Design review of the part built by this model. Coordinates are the model's own, in mm. A direction names the side the tool comes from. Give positions to 0.01 mm unless a question says otherwise; leave off trailing zeros. Loops run counter-clockwise (first coordinate to the right, second up) from the corner with the lowest first, then second, coordinate; pieces in that order, holes last. Notation, with made-up numbers: (2.25, 7.25) - (36.25, 7.25) arc R32 cw to (36.25, 42.25) - close; hole circle Ø10 at (-5, -39). An arc over 180 degrees is marked (long way). Write each question's results on one line, items separated by ' | '.
```python
from build123d import *

# Parameters (mm, degrees)
SKETCH1_W            = 31
SKETCH1_H            = 29
BOSS_EXTRUDE1_DEPTH  = 1
SKETCH2_W            = 7
SKETCH2_H            = 8
BOSS_EXTRUDE2_DEPTH  = 13
SKETCH3_W            = 7
SKETCH3_H            = 7
BOSS_EXTRUDE3_DEPTH  = 5
SKETCH4_W            = 4
SKETCH4_H            = 4
BOSS_EXTRUDE4_DEPTH  = 5
SKETCH5_R            = 2.75
CUT_EXTRUDE1_DEPTH   = 8
SKETCH6_W            = 1.591238362
SKETCH6_H            = 3.57435367
BOSS_EXTRUDE5_DEPTH  = 0.1
SKETCH7_R            = 0.879599875
BOSS_EXTRUDE6_DEPTH  = 8
FILLET2_R            = 0.5
SKETCH8_W            = 7.71
SKETCH8_H            = 5.14
BOSS_EXTRUDE7_DEPTH  = 1.5
SKETCH9_W            = 1
SKETCH9_H            = 1
BOSS_EXTRUDE8_DEPTH  = 4
SKETCH10_W           = 0.8
SKETCH10_H           = 1.5
BOSS_EXTRUDE9_DEPTH  = 0.5
SKETCH11_W           = 5
SKETCH11_H           = 4
BOSS_EXTRUDE10_DEPTH = 2
SKETCH12_W           = 0.6
SKETCH12_H           = 2.642715267
BOSS_EXTRUDE11_DEPTH = 0.5
SKETCH13_W           = 2.5
SKETCH13_H           = 2
BOSS_EXTRUDE12_DEPTH = 0.5
SKETCH14_W           = 2.401106116
SKETCH14_H           = 1.2192983
BOSS_EXTRUDE13_DEPTH = 1


with BuildPart() as part:
    # Sketch1 → Boss-Extrude1 (new body)
    with BuildSketch(Plane(origin=(0, 0, 0), x_dir=(1, 0, 0), z_dir=(0, 1, 0))):
        with Locations((15.5, 14.5)):
            Rectangle(SKETCH1_W, SKETCH1_H)
    extrude(amount=BOSS_EXTRUDE1_DEPTH)

    # Sketch2 → Boss-Extrude2 (add)
    with BuildSketch(Plane.ZY):
        with Locations((-5.5, 4)):
            Rectangle(SKETCH2_W, SKETCH2_H)
    extrude(amount=-BOSS_EXTRUDE2_DEPTH)

    # Sketch3 → Boss-Extrude3 (add)
    with BuildSketch(Plane(origin=(0, 1, 0), x_dir=(1, 0, 0), z_dir=(0, 1, 0))):
        with Locations((6.5, 13.5)):
            Rectangle(SKETCH3_W, SKETCH3_H)
    extrude(amount=BOSS_EXTRUDE3_DEPTH)

    # Sketch4 → Boss-Extrude4 (add)
    with BuildSketch(Plane(origin=(0, 6, 0), x_dir=(1, 0, 0), z_dir=(0, 1, 0))):
        with Locations((6.5, 13.5)):
            Rectangle(SKETCH4_W, SKETCH4_H)
    extrude(amount=BOSS_EXTRUDE4_DEPTH)

    # Sketch5 → Cut-Extrude1 (cut)
    with BuildSketch(Plane.ZY):
        with Locations((-5.5, 4.5)):
            Circle(SKETCH5_R)
    extrude(amount=-CUT_EXTRUDE1_DEPTH, mode=Mode.SUBTRACT)

    # Sketch6 → Boss-Extrude5 (add)
    with BuildSketch(Plane.XY.offset(-2)):
        with Locations((10.684219388, 2.787176835)):
            Rectangle(SKETCH6_W, SKETCH6_H)
    extrude(amount=BOSS_EXTRUDE5_DEPTH)

    # Sketch7 → Boss-Extrude6 (add)
    with BuildSketch(Plane.ZY.offset(-8)):
        with Locations((-5.5, 4.5)):
            Circle(SKETCH7_R)
    extrude(amount=BOSS_EXTRUDE6_DEPTH)

    # Fillet2
    fillet2_edges = [part.edges().sort_by_distance(p)[0] for p in [
        (0, 4.5, -6.379599875),
    ]]
    fillet(fillet2_edges, radius=FILLET2_R)

    # Sketch8 → Boss-Extrude7 (add)
    with BuildSketch(Plane(origin=(0, 1, 0), x_dir=(1, 0, 0), z_dir=(0, 1, 0))):
        with Locations((15.495, 24.43)):
            Rectangle(SKETCH8_W, SKETCH8_H)
        with Locations((6.785, 24.43)):
            Rectangle(SKETCH8_W, SKETCH8_H)
        with Locations((24.205, 24.43)):
            Rectangle(SKETCH8_W, SKETCH8_H)
    extrude(amount=BOSS_EXTRUDE7_DEPTH)

    # Sketch9 → Boss-Extrude8 (add)
    with BuildSketch(Plane(origin=(0, 2.5, 0), x_dir=(1, 0, 0), z_dir=(0, 1, 0))):
        with Locations((6.971468334, 25.685)):
            Rectangle(SKETCH9_W, SKETCH9_H)
        with Locations((4.431468334, 25.685)):
            Rectangle(SKETCH9_W, SKETCH9_H)
        with Locations((9.511468334, 25.685)):
            Rectangle(SKETCH9_W, SKETCH9_H)
        with Locations((4.431468334, 23.145)):
            Rectangle(SKETCH9_W, SKETCH9_H)
        with Locations((13.051468334, 23.145)):
            Rectangle(SKETCH9_W, SKETCH9_H)
        with Locations((6.971468334, 23.145)):
            Rectangle(SKETCH9_W, SKETCH9_H)
        with Locations((9.511468334, 23.145)):
            Rectangle(SKETCH9_W, SKETCH9_H)
        with Locations((18.131468334, 25.685)):
            Rectangle(SKETCH9_W, SKETCH9_H)
        with Locations((18.131468334, 23.145)):
            Rectangle(SKETCH9_W, SKETCH9_H)
        with Locations((15.591468334, 23.145)):
            Rectangle(SKETCH9_W, SKETCH9_H)
        with Locations((15.591468334, 25.685)):
            Rectangle(SKETCH9_W, SKETCH9_H)
        with Locations((13.051468334, 25.685)):
            Rectangle(SKETCH9_W, SKETCH9_H)
        with Locations((21.671468334, 23.145)):
            Rectangle(SKETCH9_W, SKETCH9_H)
        with Locations((26.751468334, 25.685)):
            Rectangle(SKETCH9_W, SKETCH9_H)
        with Locations((26.751468334, 23.145)):
            Rectangle(SKETCH9_W, SKETCH9_H)
        with Locations((24.211468334, 23.145)):
            Rectangle(SKETCH9_W, SKETCH9_H)
        with Locations((24.211468334, 25.685)):
            Rectangle(SKETCH9_W, SKETCH9_H)
        with Locations((21.671468334, 25.685)):
            Rectangle(SKETCH9_W, SKETCH9_H)
    extrude(amount=BOSS_EXTRUDE8_DEPTH)

    # Sketch10 → Boss-Extrude9 (add)
    with BuildSketch(Plane(origin=(0, 1, 0), x_dir=(1, 0, 0), z_dir=(0, 1, 0))):
        with Locations((18.786083485, 18.300770285)):
            Rectangle(SKETCH10_W, SKETCH10_H)
        with Locations((14.786083485, 18.300770285)):
            Rectangle(SKETCH10_W, SKETCH10_H)
        with Locations((22.786083485, 18.300770285)):
            Rectangle(SKETCH10_W, SKETCH10_H)
        with Locations((26.786083485, 18.300770285)):
            Rectangle(SKETCH10_W, SKETCH10_H)
    extrude(amount=BOSS_EXTRUDE9_DEPTH)

    # Sketch11 → Boss-Extrude10 (add)
    with BuildSketch(Plane(origin=(0, 1, 0), x_dir=(1, 0, 0), z_dir=(0, 1, 0))):
        with Locations((25.443805994, 10.374755585)):
            Rectangle(SKETCH11_W, SKETCH11_H)
        with Locations((18.443805994, 10.374755585)):
            Rectangle(SKETCH11_W, SKETCH11_H)
    extrude(amount=BOSS_EXTRUDE10_DEPTH)

    # Sketch12 → Boss-Extrude11 (add)
    with BuildSketch(Plane(origin=(0, 1, 0), x_dir=(1, 0, 0), z_dir=(0, 1, 0))):
        with Locations((17.095277575, 13.696113219)):
            Rectangle(SKETCH12_W, SKETCH12_H)
        with Locations((24.095277575, 13.696113219)):
            Rectangle(SKETCH12_W, SKETCH12_H)
        with Locations((18.365277575, 13.696113219)):
            Rectangle(SKETCH12_W, SKETCH12_H)
        with Locations((19.635277575, 13.696113219)):
            Rectangle(SKETCH12_W, SKETCH12_H)
        with Locations((25.365277575, 13.696113219)):
            Rectangle(SKETCH12_W, SKETCH12_H)
        with Locations((26.635277575, 13.696113219)):
            Rectangle(SKETCH12_W, SKETCH12_H)
    extrude(amount=BOSS_EXTRUDE11_DEPTH)

    # Sketch13 → Boss-Extrude12 (add)
    with BuildSketch(Plane(origin=(0, 1, 0), x_dir=(1, 0, 0), z_dir=(0, 1, 0))):
        with Locations((18.365277575, 7.374755585)):
            Rectangle(SKETCH13_W, SKETCH13_H)
        with Locations((25.365277575, 7.374755585)):
            Rectangle(SKETCH13_W, SKETCH13_H)
    extrude(amount=BOSS_EXTRUDE12_DEPTH)

    # Sketch14 → Boss-Extrude13 (add)
    with BuildSketch(Plane(origin=(0, 1, 0), x_dir=(1, 0, 0), z_dir=(0, 1, 0))):
        with Locations((23.540566393, 4.488126974)):
            Rectangle(SKETCH14_W, SKETCH14_H)
        with Locations((18.540566393, 4.488126974)):
            Rectangle(SKETCH14_W, SKETCH14_H)
        with Locations((23.540566393, 1.988126974)):
            Rectangle(SKETCH14_W, SKETCH14_H)
        with Locations((18.540566393, 1.988126974)):
            Rectangle(SKETCH14_W, SKETCH14_H)
    extrude(amount=BOSS_EXTRUDE13_DEPTH)


solid = part.part
```
Item 1: We need section A-A on z = -16.5. Give the boundary of the cut face in (x, y).
Output values:
outline: (0, 0) - (31, 0) - (31, 1) - (10, 1) - (10, 6) - (3, 6) - (3, 1) - (0, 1) - close
Item 2: We need section D-D on z = -7. Give the boundary of the cut face in (x, y), then the cut area to 3 significant figures.
Output values:
outline: (0, 0) - (31, 0) - (31, 1) - (26.62, 1) - (26.62, 1.5) - (24.12, 1.5) - (24.12, 1) - (19.62, 1) - (19.62, 1.5) - (17.12, 1.5) - (17.12, 1) - (13, 1) - (13, 8) - (0, 8) - (0, 6.8) - (8, 6.8) - (8, 2.2) - (0, 2.2) - close | area: 87.6 mm²
Item 3: We need section C-C on z = -10.5. Give the boundary of the cut face in (x, y), then the cut area to 3 significant figures.
Output values:
outline: (0, 0) - (31, 0) - (31, 1) - (27.94, 1) - (27.94, 3) - (22.94, 3) - (22.94, 1) - (20.94, 1) - (20.94, 3) - (15.94, 3) - (15.94, 1) - (10, 1) - (10, 6) - (3, 6) - (3, 1) - (0, 1) - close | area: 86.0 mm²
Item 4: Wall thickness on probe 1 along Y at (x, z) = (5, -5.5); probe 2 along X at (y, z) = (1.75, -5); probe 3 along Z at (x, y) = (18.5, 5.75) (3 decimals): over which ranges is each line inside the solid? List them lowest first.
Output values:
probe 1: y = 0 to 1.75, 3.62 to 5.38, 7.25 to 8 | probe 2: x = 0 to 13, 17.34 to 19.74, 22.34 to 24.74 | probe 3: z = -26.185 to -25.185, -23.645 to -22.645
Item 5: Clearance check with flat-ended pins moving along their axes: P1, Ø0.5, axis at x = 22, z = -25.5, coming from the +Y side; P2, Ø0.5, axis at x = 15.5, y = 4, coming from the -Z side (3 decimals); P3, Ø6, axis at x = 14.5, z = -15.5, coming from the +Y side. State where each tip first meets the part, or that it passes through.
Output values:
P1: stops at y = 6.5 | P2: stops at z = -26.185 | P3: stops at y = 1.5
Item 6: Draft analysis for pull direction X (two halves, no side actions). For faces 4 (the face through (17.631, 4, -26)), 5 (the face through (15.6, 4.5, -23.645)), state which applies: +X half, -X half, draft (parallel to the pull), parting line (faces both ways), or undercut.
Output values:
face 4: undercut | face 5: draft
Item 7: Tool access review of faces 1 (the face through (18.5, 1.5, -1.378)), 2 (the face through (6, 4, -9)), 3 (the face through (9.5, 4.5, -22.645)): name each direction out of +Z, -Z, +X, -X, +Y, -Y from which nothing blocks a thin tool from reaching the whole face with its end or side.
Output values:
face 1: +Z, +X, -X, +Y | face 2: -X, +Y | face 3: +X, -X, +Y
Item 8: We need section B-B on y = 10. Give the boundary of the cut face in (x, z), then the cut area to 3 significant figures.
Output values:
outline: (4.5, -15.5) - (8.5, -15.5) - (8.5, -11.5) - (4.5, -11.5) - close | area: 16.0 mm²
